```python
from build123d import *

# Parameters (mm, degrees)
SKETCH_W        = 9.5
SKETCH_H        = 17
PAD_DEPTH       = 39
SKETCH001_W     = 9.5
SKETCH001_H     = 26
POCKET_DEPTH    = 5
SKETCH002_W     = 1.9
SKETCH002_H     = 24
POCKET001_DEPTH = 17
COPYSKETCH003_W = 9.5
COPYSKETCH003_H = 24
POCKET002_DEPTH = 7


with BuildPart() as part:
    # Sketch → Pad (new body)
    with BuildSketch(Plane.XY):
        with Locations((0, 8.5)):
            Rectangle(SKETCH_W, SKETCH_H)
    extrude(amount=PAD_DEPTH)

    # Sketch001 (on Face3 of Pad) → Pocket (cut)
    with BuildSketch(Plane.XZ):
        with Locations((0, 13)):
            Rectangle(SKETCH001_W, SKETCH001_H)
    extrude(amount=-POCKET_DEPTH, mode=Mode.SUBTRACT)

    # Sketch002 (on Face1 of Pocket) → Pocket001 (cut)
    with BuildSketch(Plane(origin=(0, 17, 0), x_dir=(-1, 0, 0), z_dir=(0, 1, 0))):
        with Locations((-3.8, 12)):
            Rectangle(SKETCH002_W, SKETCH002_H)
        with Locations((3.8, 12)):
            Rectangle(SKETCH002_W, SKETCH002_H)
    extrude(amount=-POCKET001_DEPTH, mode=Mode.SUBTRACT)

    # CopySketch003 → Pocket002 (cut)
    with BuildSketch(Plane.XZ):
        with Locations((0, 12)):
            Rectangle(COPYSKETCH003_W, COPYSKETCH003_H)
    extrude(amount=-POCKET002_DEPTH, mode=Mode.SUBTRACT)


solid = part.part
```
Geometry: final body of the model. Coordinates: model frame, mm. A direction names the side the tool comes from. Coordinates: 2 decimals unless noted, no trailing zeros. Loops run counter-clockwise (first coordinate to the right, second up) from the corner with the lowest first, then second, coordinate; pieces in that order, holes last. Notation, with made-up numbers: (-12, 88.25) -> (41, 88.25) arc R20 cw to (41, 98.25) -> close; hole circle Ø6 at (54, 69). An arc over 180 degrees is marked (long way). Use a Markdown table: item, result. Add a question column.
(1) Section query A-A, the plane x = -2. Return loops of the section in (y, z), plus the area to 3 significant figures.
(2) Pin query (flat end, axial travel): pin 1 Ø5 at (y, z) = (11.5, 13) entering from -X; pin 2 Ø8 at (y, z) = (13.5, 7) entering from +X; pin 3 Ø1.5 at (x, y) = (1, 1.5) entering from -Z. Return the tip coordinate at first contact, or that it passes through.
(3) Section query D-D, the plane y = 4.5. Return loops of the section in (x, z), plus the area to 4 significant figures.
(4) Section query C-C, the plane z = 25.5. Return loops of the section in (x, y), plus the area to 3 significant figures.
(5) Access query for faces 1 (the flat face through (2.85, 12, 12)), 2 (the flat face through (-2.85, 12, 12)), 3 (the flat face through (0, 5, 25)). Directions: +Z, -Z, +X, -X, +Y, -Y. A direction counts if a zero-diameter tool reaches every point of the face in a straight line with its end or side. Return the directions, or none.
(6) Section query B-B, the plane y = 10. Return loops of the section in (x, z).
(7) Line query: line 1 along Y through (x, z) = (1.75, 11.5); line 2 along X through (y, z) = (12.75, 10.5); line 3 along Z through (x, y) = (-2, 4). Output: solid intervals per line, ascending.
Answer:
| question | item | result |
|---|---|---|
| 1 | outline | (0, 26) -> (5, 26) -> (5, 24) -> (7, 24) -> (7, 0) -> (17, 0) -> (17, 39) -> (0, 39) -> close |
| 1 | area | 485 mm^2 |
| 2 | pin 1 | stops at x = -2.85 |
| 2 | pin 2 | stops at x = 2.85 |
| 2 | pin 3 | stops at z = 26 |
| 3 | outline | (-4.75, 26) -> (4.75, 26) -> (4.75, 39) -> (-4.75, 39) -> close |
| 3 | area | 123.5 mm^2 |
| 4 | outline | (-4.75, 5) -> (4.75, 5) -> (4.75, 17) -> (-4.75, 17) -> close |
| 4 | area | 114 mm^2 |
| 5 | face 1 | -Z, +X, +Y, -Y |
| 5 | face 2 | -Z, -X, +Y, -Y |
| 5 | face 3 | -Z, +X, -X, -Y |
| 6 | outline | (-4.75, 24) -> (-2.85, 24) -> (-2.85, 0) -> (2.85, 0) -> (2.85, 24) -> (4.75, 24) -> (4.75, 39) -> (-4.75, 39) -> close |
| 7 | line 1 | y = 7 to 17 |
| 7 | line 2 | x = -2.85 to 2.85 |
| 7 | line 3 | z = 26 to 39 |
